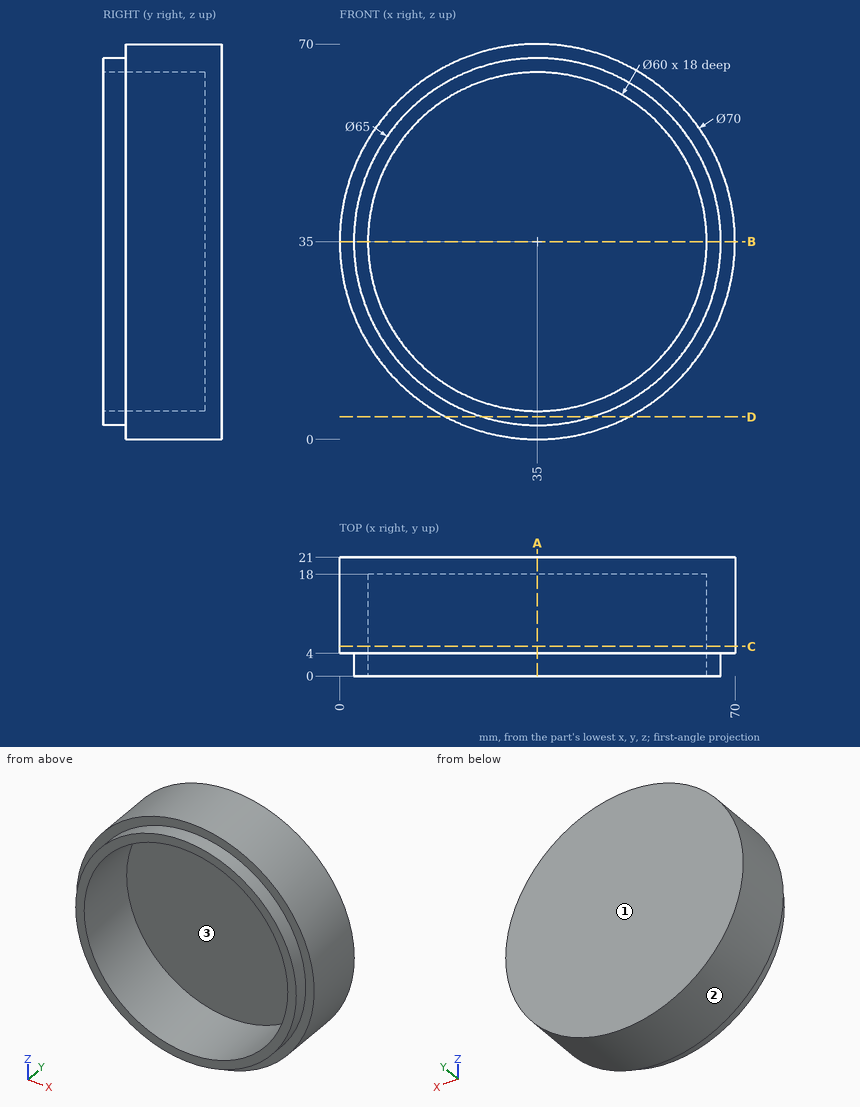
Drawing for the job (mm, zero at the part's lowest x, y, z). Give positions to 0.01 mm unless a question says otherwise; leave off trailing zeros. Write each loop counter-clockwise with the first axis right and the second up, starting at its lowest first coordinate (ties: lowest second). Pieces come first, ordered by that corner, then holes. Notation, with made-up numbers: M 86,29 L 134,29 A7 ccw 134,39 Z; hole C 67.25,87.25 d11. An arc over 180 degrees is marked long. Return JSON: item names as keys, results as strings. Group by question number.
(1) Band-saw the part on D-D (z = 4). Give the cut face in (x, y).
(2) Mould opens along X. For the marked faces 1, 2 and 3 say: pulls with the +X half, pulls with the -X half, needs draft (parallel to the pull), parting line crosses it, or undercut.
(3) Drill centre lines: L1, parallel to Z at x = 35, y = 13.5; L2, parallel to Y at x = 29.5, z = 50; L3, parallel to Z at x = 33, y = 9.75. Where is each one in solid material? Low to high. Write a range as [from, to].
(4) Flat gauge pins, fed straight in: pin 1 Ø4 at (y, z) = (16.5, 12) entering from +X; pin 2 Ø3 at (x, z) = (51, 19.5) entering from -Y; pin 3 Ø5 at (x, y) = (24, 8.5) entering from -Z. Where does each tip first touch, or does it go through?
(5) Band-saw the part on C-C (y = 5.25). Give the cut face in (x, z), and give its area (3 significant figures).
(6) Band-saw the part on B-B (z = 35). Give the cut face in (x, y), and give its area (3 significant figures).
(7) Band-saw the part on A-A (x = 35). Give the cut face in (y, z), and give its area (3 significant figures).
Entries:
{
 "1": {"outline": "M 18.75,4 L 25.24,4 L 25.24,0 L 44.76,0 L 44.76,4 L 51.25,4 L 51.25,21 L 18.75,21 Z"},
 "2": {"face 1": "needs draft", "face 2": "parting line crosses it", "face 3": "undercut"},
 "3": {"L1": "z = [0, 5], [65, 70]", "L2": "y = [18, 21]", "L3": "z = [0.06, 5.07], [64.93, 69.94]"},
 "4": {"pin 1": "stops at x = 63", "pin 2": "stops at y = 18", "pin 3": "stops at z = 1.05"},
 "5": {"outline": "C 35,35 d70; hole C 35,35 d60", "area": "1,020 mm^2"},
 "6": {"outline": "M 0,4 L 2.5,4 L 2.5,0 L 5,0 L 5,18 L 65,18 L 65,0 L 67.5,0 L 67.5,4 L 70,4 L 70,21 L 0,21 Z", "area": "370 mm^2"},
 "7": {"outline": "M 0,2.5 L 4,2.5 L 4,0 L 21,0 L 21,70 L 4,70 L 4,67.5 L 0,67.5 L 0,65 L 18,65 L 18,5 L 0,5 Z", "area": "370 mm^2"}
}
